CAD build for the part. Positions are in the model's coordinates, mm. A direction names the side the tool comes from. Coordinates: 2 decimals unless noted, no trailing zeros. Write each loop counter-clockwise with the first axis right and the second up, starting at its lowest first coordinate (ties: lowest second). Pieces come first, ordered by that corner, then holes.
Autodesk Inventor part; units mm, degrees
ref_plane "YZ Plane" through (0, 0, 0) normal (1, 0, 0) x (0, 1, 0)
ref_plane "XZ Plane" through (0, 0, 0) normal (0, 1, 0) x (-1, 0, 0)
ref_plane "XY Plane" through (0, 0, 0) normal (0, 0, 1) x (1, 0, 0)
sketch "Sketch1" plane through (0, 0, 0) normal (0, 0, 1) x (1, 0, 0)
  line L0 (0, 0) -> (25.4, 0)
  line L1 (25.4, 0) -> (25.4, 50.8)
  line L2 (25.4, 50.8) -> (0, 50.8)
  line L3 (0, 50.8) -> (0, 0)
  line L4 (23.8125, 49.2125) -> (23.8125, 1.5875)
  line L5 (23.8125, 1.5875) -> (1.5875, 1.5875)
  line L6 (1.5875, 1.5875) -> (1.5875, 49.2125)
  line L7 (1.5875, 49.2125) -> (23.8125, 49.2125)
  dimension "d0" = 25.4
  dimension "d1" = 50.8
  dimension "d2" = 1.5875
extrude "Extrusion1" add sketch "Sketch1" along normal blind 762
sketch "Sketch2" plane through (0, 0, 0) normal (0, -1, 0) x (1, 0, 0)
  line L0 (1.5875, 762) -> (23.8125, 762) construction
  line L1 (12.7, 762) -> (12.7, 646.6078) construction
  line L2 (12.7, 646.6078) -> (12.7, 526.6182) construction
  line L3 (12.7, 526.6182) -> (12.7, 406.6286) construction
  line L4 (12.7, 406.6286) -> (12.7, 286.639) construction
  line L5 (12.7, 286.639) -> (12.7, 166.6494) construction
  line L6 (23.8125, 0) -> (1.5875, 0) construction
  line L7 (12.7, 0) -> (12.7, 12.7) construction
  line L8 (12.7, 12.7) -> (12.7, 38.1) construction
  line L9 (12.7, 38.1) -> (12.7, 63.5) construction
  line L10 (12.7, 63.5) -> (12.7, 88.9) construction
  circle A0 centre (12.7, 12.7) radius 2.5797
  circle A1 centre (12.7, 38.1) radius 2.5797
  circle A2 centre (12.7, 63.5) radius 2.5797
  circle A3 centre (12.7, 166.6494) radius 2.5797
  circle A4 centre (12.7, 286.639) radius 2.5797
  circle A5 centre (12.7, 406.6286) radius 2.5797
  circle A6 centre (12.7, 526.6182) radius 2.5797
  point P0 (0, 0)
  dimension "d5" = 115.3922
  dimension "d6" = 119.9896
  dimension "d7" = 119.9896
  dimension "d8" = 119.9896
  dimension "d9" = 119.9896
  dimension "d10" = 12.7
  dimension "d11" = 25.4
  dimension "d12" = 25.4
  dimension "d13" = 25.4
  dimension "d14" = 5.1594
  dimension "d15" = 5.1594
  dimension "d16" = 5.1594
  dimension "d18" = 5.1594
  dimension "d19" = 5.1594
  dimension "d20" = 5.1594
  dimension "d21" = 5.1594
sketch "Sketch3" plane through (0, 50.8, 0) normal (0, 1, 0) x (1, 0, 0)
  line L0 (0, -762) -> (25.4, -762) construction
  line L1 (12.7, -762) -> (12.7, -749.3) construction
  circle A0 centre (12.7, -749.3) radius 2.5797
  point P0 (0, 0)
  dimension "d27" = 12.7
  dimension "d28" = 5.1594
extrude "Extrusion4" cut sketch "Sketch3" against normal blind 525.4625
sketch "Sketch6" plane through (0, 50.8, 0) normal (0, 1, 0) x (1, 0, 0)
  line L0 (0, -762) -> (25.4, -762) construction
  line L1 (12.7, -762) -> (12.7, -673.1) construction
  line L2 (12.7, -673.1) -> (12.7, -698.5) construction
  line L3 (12.7, -698.5) -> (12.7, -647.7) construction
  circle A0 centre (12.7, -698.5) radius 2.5797
  circle A1 centre (12.7, -673.1) radius 2.5797
  circle A2 centre (12.7, -647.7) radius 2.5797
  point P0 (0, 0)
  dimension "d53" = 88.9
  dimension "d54" = 25.4
  dimension "d55" = 50.8
  dimension "d56" = 5.1594
  dimension "d61" = 5.1594
  dimension "d62" = 5.1594
extrude "Extrusion7" cut sketch "Sketch6" against normal blind 107.95
extrude "Extrusion8" cut sketch "Sketch2" against normal blind 107.95
sketch "Sketch7" plane through (25.4, 0, 0) normal (1, 0, 0) x (0, 0, -1)
  line L0 (-762, 50.8) -> (-762, 0)
  line L1 (-762, 25.4) -> (-711.2, 25.4) construction
  line L2 (-711.2, 25.4) -> (-635, 25.4) construction
  line L3 (-635, 25.4) -> (-711.2, 25.4) construction
  line L4 (-649.2875, 39.6875) -> (-696.9125, 39.6875)
  line L5 (-696.9125, 11.1125) -> (-649.2875, 11.1125)
  arc A0 (-649.2875, 11.1125) -> (-649.2875, 39.6875) centre (-649.2875, 25.4) ccw
  arc A1 (-696.9125, 39.6875) -> (-696.9125, 11.1125) centre (-696.9125, 25.4) ccw
  point P0 (0, 0)
  point P1 (-673.1, 25.4)
  dimension "d63" = 50.8
  dimension "d64" = 76.2
  dimension "d65" = 28.575
extrude "Extrusion9" cut sketch "Sketch7" against normal blind 25.4
sketch "Sketch8" plane through (0, 50.8, 0) normal (0, 1, 0) x (1, 0, 0)
  line L0 (0, -762) -> (25.4, -762) construction
  line L1 (12.7, -762) -> (12.7, -723.9) construction
  circle A0 centre (12.7, -723.9) radius 2.5797
  line L2 (0, 0) -> (25.4, 0) construction
  line L3 (12.7, 0) -> (12.7, -88.9) construction
  circle A1 centre (12.7, -88.9) radius 2.5797
  dimension "d68" = 38.1
  dimension "d69" = 5.1594
  dimension "d72" = 88.9
extrude "Extrusion11" cut sketch "Sketch8" against normal blind 50.8
properties part number "1x2 30in"
Item 1: Flat gauge pin, fed straight in: pin 1 Ø5 at (x, y) = (6.5, 42.5) entering from -Z. Where does the tip first touch, or does it go through?
Item 2: Saw through at A-A, the plane y = 25.4. Write the cut outline in (x, z), and give its area (3 significant figures).
Item 3: Wall check: line 1 along Y through (x, z) = (5, 506); line 2 along X through (y, z) = (29.5, 186.5); line 3 along X through (y, z) = (50.2, 698.5). Give the ranges that are in metal, low to high.
Item 4: Which spindle directions (+Z, -Z, +X, -X, +Y, -Y) get a long thin tool onto all of the face, cutting with end or side? Do faces 1 (the flat face through (23.812, 26, 376)), 2 (the flat face through (13, 0, 376)), 3 (the cylindrical face through (24.617, 25.086, 635.003)). Say none if no direction does.
Item 5: Saw through at B-B, the plane z = 264. Write the cut outline in (x, y), and give its area (3 significant figures).
Item 6: Two-plate mould, pull along Z, no slides. Class faces 4 (the flat face through (13, 50.8, 376)), 5 (the cylindrical face through (24.617, 25.714, 711.197)), 6 (the flat face through (1, 27, 762)), 7 (the flat face through (1, 27, 0)): +Z half, -Z half, draft (parallel to the pull), parting line (faces both ways), or undercut.
Working result:
1. pin 1: passes through
2. outline: (0, 0) - (1.59, 0) - (1.59, 635) - (0, 635) - close; (0, 711.2) - (1.59, 711.2) - (1.59, 762) - (0, 762) - close; (23.81, 0) - (25.4, 0) - (25.4, 635) - (23.81, 635) - close; (23.81, 711.2) - (25.4, 711.2) - (25.4, 762) - (23.81, 762) - close
2. area: 2,180 mm2
3. line 1: y = 0 to 1.59, 49.21 to 50.8
3. line 2: x = 0 to 1.59, 23.81 to 25.4
3. line 3: x = 0 to 10.12, 15.28 to 25.4
4. face 1: +Z, -Z
4. face 2: +Z, -Z, +X, -X, -Y
4. face 3: +X, -X
5. outline: (0, 0) - (25.4, 0) - (25.4, 50.8) - (0, 50.8) - close; hole (1.59, 1.59) - (23.81, 1.59) - (23.81, 49.21) - (1.59, 49.21) - close
5. area: 232 mm2
6. face 4: draft
6. face 5: undercut
6. face 6: +Z half
6. face 7: -Z half
